Build history of the part. All positions in model axes, mm. Face numbers are marked on the shaded views. A direction names the side the tool comes from. Round coordinates to 2 decimals unless told otherwise and drop trailing zeros. Write each loop counter-clockwise with the first axis right and the second up, starting at its lowest first coordinate (ties: lowest second). Pieces come first, ordered by that corner, then holes.
Item 1: Drop flat-ended pins along their axis: pin 1 Ø2.5 at (y, z) = (-8, 50) entering from +X; pin 2 Ø7 at (x, y) = (-10, -8) entering from +Z; pin 3 Ø8 at (x, y) = (11, -8.5) entering from +Z; pin 4 Ø8 at (y, z) = (-7.5, 46) entering from -X. Give the stop position or say it passes through.
Item 2: Band-saw the part on A-A, the plane y = -8. Write the cut outline in (x, z).
Item 3: 3-axis set-ups, long thin cutter, end or side, ignore diameter. For the marked faces 1, 2, 3, 4 and 5: which of +Z, -Z, +X, -X, +Y, -Y reach the whole face in a straight line?
Item 4: Wall check: probe 1 along Z at (x, y) = (1.6, -8); probe 2 along Z at (x, y) = (18, -14.25); probe 3 along Y at (x, z) = (-10, -1.1). Give the ranges that are in metal, low to high.
Item 5: Band-saw the part on B-B, the plane x = 49. Write the cut outline in (y, z), then the cut area to 3 significant figures.
Item 6: Band-saw the part on C-C, the plane z = 50. Write the cut outline in (x, y), then the cut area to 3 significant figures.
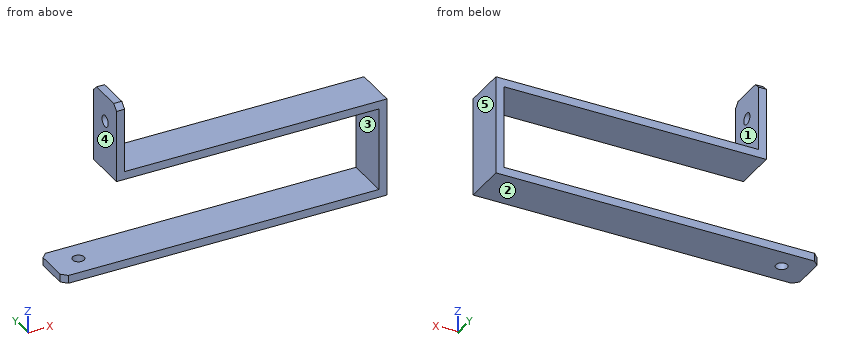
```python
from build123d import *

# Parameters (mm, degrees)
F1_DEPTH = 16
F2_R     = 2.15
F3_DEPTH = 25
F4_R     = 2.15
F5_DEPTH = 25
F6_SIZE  = 2


with BuildPart() as f1:
    # F0 (on Front) → F1 (new body)
    with BuildSketch(Plane.XZ):
        Polygon((98, 0), (0, 0), (-20, 0), (-20, -3), (0, -3), (101, -3), (101, 34), (3, 34), (3, 60), (0, 60), (0, 31), (98, 31), align=None)
    extrude(amount=F1_DEPTH)

    # F2 (on face) → F3 (cut)
    with BuildSketch(Plane.XY):
        with Locations((-10, -8)):
            Circle(F2_R)
    extrude(amount=-F3_DEPTH, mode=Mode.SUBTRACT)

    # F4 (on face) → F5 (cut)
    with BuildSketch(Plane(origin=(0, 0, 0), x_dir=(0, -1, 0), z_dir=(-1, 0, 0))):
        with Locations((8, 50)):
            Circle(F4_R)
    extrude(amount=-F5_DEPTH, mode=Mode.SUBTRACT)

    # F6
    f6_edges = [f1.edges().sort_by_distance(p)[0] for p in [
        (1.5, -16, 60),
        (1.5, 0, 60),
        (-20, -16, -1.5),
        (-20, 0, -1.5),
    ]]
    chamfer(f6_edges, length=F6_SIZE)


solid = f1.part
```
Results:
1. pin 1: passes through
1. pin 2: stops at z = 0
1. pin 3: stops at z = 34
1. pin 4: stops at x = 0
2. outline: (-20, -3) - (-12.15, -3) - (-12.15, 0) - (-20, 0) - close; (-7.85, -3) - (101, -3) - (101, 34) - (3, 34) - (3, 47.85) - (0, 47.85) - (0, 31) - (98, 31) - (98, 0) - (-7.85, 0) - close; (0, 52.15) - (3, 52.15) - (3, 60) - (0, 60) - close
3. face 1: +Z, +X, +Y, -Y
3. face 2: -Z, +X, -X, +Y, -Y
3. face 3: -X, +Y, -Y
3. face 4: +Z, -X, +Y, -Y
3. face 5: +Z, -Z, +X, +Y, -Y
4. probe 1: z = -3 to 0, 31 to 47.85, 52.15 to 60
4. probe 2: z = -3 to 0, 31 to 34
4. probe 3: y = -16 to -10.15, -5.85 to 0
5. outline: (-16, -3) - (0, -3) - (0, 0) - (-16, 0) - close; (-16, 31) - (0, 31) - (0, 34) - (-16, 34) - close
5. area: 96.0 mm2
6. outline: (0, -16) - (3, -16) - (3, -10.15) - (0, -10.15) - close; (0, -5.85) - (3, -5.85) - (3, 0) - (0, 0) - close
6. area: 35.1 mm2
